```python
from build123d import *

# Parameters (mm, degrees)
F1_DEPTH = 127
F4_DEPTH = 45.72
F5_R     = 2.54
F6_R     = 4.7625
F7_DEPTH = 11.557


with BuildPart() as f1:
    # F0 (on Front) → F1 (new body)
    with BuildSketch(Plane.XZ):
        with BuildLine():
            Line((0, 57.277), (0, 0))
            Line((0, 0), (12.7, 0))
            ThreePointArc((12.7, 0), (50.927, 38.227), (89.154, 0))
            Line((89.154, 0), (101.854, 0))
            Line((101.854, 0), (101.854, 57.277))
            Line((101.854, 57.277), (0, 57.277))
        make_face()
    extrude(amount=F1_DEPTH)

    # F3 (on face) → F4 (cut)
    with BuildSketch(Plane(origin=(0, 0, 0), x_dir=(1, 0, 0), z_dir=(0, 0, -1))):
        Polygon((50.927, 123.825), (3.175, 123.825), (3.175, 3.175), (50.927, 3.175), (98.679, 3.175), (98.679, 123.825), align=None)
    extrude(amount=-F4_DEPTH, mode=Mode.SUBTRACT)

    # F5
    f5_edges = [f1.edges().sort_by_distance(p)[0] for p in [
        (3.175, -63.5, 45.72),
        (98.679, -63.5, 45.72),
        (50.927, -123.825, 45.72),
        (98.679, -123.825, 22.86),
        (3.175, -123.825, 22.86),
        (98.679, -3.175, 22.86),
        (50.927, -3.175, 45.72),
        (3.175, -3.175, 22.86),
    ]]
    fillet(f5_edges, radius=F5_R)

    # F6 (on face) → F7 (cut, through all)
    with BuildSketch(Plane(origin=(0, 0, 45.72), x_dir=(1, 0, 0), z_dir=(0, 0, -1))):
        with Locations((50.927, 95.885)):
            Circle(F6_R)
        with Locations((50.927, 31.115)):
            Circle(F6_R)
    extrude(amount=-F7_DEPTH, mode=Mode.SUBTRACT)


solid = f1.part
```
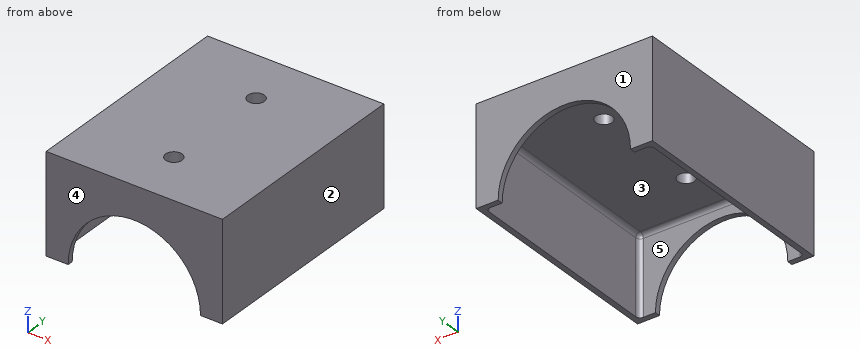
The model under review builds one solid part; all positions refer to its coordinate system, in mm. Face numbers are marked on the shaded views. A direction names the side the tool comes from. Round coordinates to 2 decimals unless told otherwise and drop trailing zeros. Loops run counter-clockwise (first coordinate to the right, second up) from the corner with the lowest first, then second, coordinate; pieces in that order, holes last. Notation, with made-up numbers: (10, 23.25) - (43, 23.25) arc R34 cw to (43, 56.25) - close; hole circle Ø4 at (24, -32.5). An arc over 180 degrees is marked (long way). Use a Markdown table: item, result. Add a question column.
Q1. Add section B-B (z = 33). State the section outline as (x, y) points (3 decimals).
Q2. Add section C-C (y = -38.5). State the section outline as (x, z) points (3 decimals).
Q3. Add section D-D (x = 31). State the section outline as (y, z) points (3 decimals).
Q4. Add section A-A (x = 51). State the section outline as (y, z) points (3 decimals), plus the area to 3 significant figures.
Q5. Insertion check: pin 1 Ø6 at (x, y) = (50.5, -17) entering from -Z; pin 2 Ø21.5 at (x, z) = (38.5, 15) entering from +Y. Each pin has a flat end and moves straight along its axis. Give the tip position at first contact, or say it passes through.
Q6. For probe 1 along Y at (x, z) = (34, 43) (3 decimals); probe 2 along X at (y, z) = (-32.5, 35) (3 decimals); probe 3 along Z at (x, y) = (13.5, -33), list the stretches that pass through material, from the lowest coordinate up.
Q7. The part is to be moulded in two halves that separate along Y. For the marked faces 1, 2 and 3, say which applies: pulls with the +Y half, pulls with the -Y half, needs draft (parallel to the pull), parting line crosses it, or undercut.
Q8. Machinability: for the marked faces 4 and 5, which of the approach directions +Z, -Z, +X, -X, +Y, -Y give a long, thin tool a straight path to every point of the face, cutting with its end or side? Answer none if there is none.
Worked answers:
| question | item | result |
|---|---|---|
| 1 | outline | (0, -127) - (31.632, -127) - (31.632, -123.825) - (5.715, -123.825) arc R2.54 cw to (3.175, -121.285) - (3.175, -5.715) arc R2.54 cw to (5.715, -3.175) - (31.632, -3.175) - (31.632, 0) - (0, 0) - close; (70.222, -127) - (101.854, -127) - (101.854, 0) - (70.222, 0) - (70.222, -3.175) - (96.139, -3.175) arc R2.54 cw to (98.679, -5.715) - (98.679, -121.285) arc R2.54 cw to (96.139, -123.825) - (70.222, -123.825) - close |
| 2 | outline | (0, 0) - (3.175, 0) - (3.175, 43.18) arc R2.54 cw to (5.715, 45.72) - (96.139, 45.72) arc R2.54 cw to (98.679, 43.18) - (98.679, 0) - (101.854, 0) - (101.854, 57.277) - (0, 57.277) - close |
| 3 | outline | (-127, 32.622) - (-123.825, 32.622) - (-123.825, 43.18) arc R2.54 cw to (-121.285, 45.72) - (-5.715, 45.72) arc R2.54 cw to (-3.175, 43.18) - (-3.175, 32.622) - (0, 32.622) - (0, 57.277) - (-127, 57.277) - close |
| 4 | outline | (-127, 38.227) - (-123.825, 38.227) - (-123.825, 43.18) arc R2.54 cw to (-121.285, 45.72) - (-100.647, 45.72) - (-100.647, 57.277) - (-127, 57.277) - close; (-91.123, 45.72) - (-35.877, 45.72) - (-35.877, 57.277) - (-91.123, 57.277) - close; (-26.353, 45.72) - (-5.715, 45.72) arc R2.54 cw to (-3.175, 43.18) - (-3.175, 38.227) - (0, 38.227) - (0, 57.277) - (-26.353, 57.277) - close |
| 4 | area | 1,300 mm² |
| 5 | pin 1 | z = 45.72 |
| 5 | pin 2 | through |
| 6 | probe 1 | -127 to -123.825, -3.175 to 0 |
| 6 | probe 2 | 0 to 3.175, 98.679 to 101.854 |
| 6 | probe 3 | 45.72 to 57.28 |
| 7 | face 1 | pulls with the +Y half |
| 7 | face 2 | needs draft |
| 7 | face 3 | undercut |
| 8 | face 4 | +Z, -Z, +X, -X, -Y |
| 8 | face 5 | -Z |
